from build123d import *

# Parameters (mm, degrees)
SKETCH_1_W      = 10.3
SKETCH_1_H      = 10.3
EXTRUDE_1_DEPTH = 100


with BuildPart() as part:
    # 草图1 → 凸台-拉伸1 (new body)
    with BuildSketch(Plane.XY):
        with BuildLine():
            Line((-3.371587854, 9.357012623), (-6.271587854, 9.357012623))
            Line((-6.271587854, 9.357012623), (-6.271587854, 17.757012623))
            Line((-6.271587854, 17.757012623), (-3.871587854, 17.757012623))
            ThreePointArc((-3.871587854, 17.757012623), (-3.518034464, 17.903459232), (-3.371587854, 18.257012623))
            Line((-3.371587854, 18.257012623), (-3.371587854, 20.257012623))
            ThreePointArc((-3.371587854, 20.257012623), (-3.518034464, 20.610566013), (-3.871587854, 20.757012623))
            Line((-3.871587854, 20.757012623), (-18.771587854, 20.757012623))
            ThreePointArc((-18.771587854, 20.757012623), (-19.125141245, 20.610566013), (-19.271587854, 20.257012623))
            Line((-19.271587854, 20.257012623), (-19.271587854, 5.357012623))
            ThreePointArc((-19.271587854, 5.357012623), (-19.125141245, 5.003459232), (-18.771587854, 4.857012623))
            Line((-18.771587854, 4.857012623), (-16.771587854, 4.857012623))
            ThreePointArc((-16.771587854, 4.857012623), (-16.418034464, 5.003459232), (-16.271587854, 5.357012623))
            Line((-16.271587854, 5.357012623), (-16.271587854, 7.757012623))
            Line((-16.271587854, 7.757012623), (-7.871587854, 7.757012623))
            Line((-7.871587854, 7.757012623), (-7.871587854, 4.857012623))
            Line((-7.871587854, 4.857012623), (-6.641587854, 6.087012623))
            Line((-6.641587854, 6.087012623), (-6.641587854, -4.572987377))
            Line((-6.641587854, -4.572987377), (-7.871587854, -3.342987377))
            Line((-7.871587854, -3.342987377), (-7.871587854, -6.242987377))
            Line((-7.871587854, -6.242987377), (-16.271587854, -6.242987377))
            Line((-16.271587854, -6.242987377), (-16.271587854, -3.842987377))
            ThreePointArc((-16.271587854, -3.842987377), (-16.418034464, -3.489433987), (-16.771587854, -3.342987377))
            Line((-16.771587854, -3.342987377), (-18.771587854, -3.342987377))
            ThreePointArc((-18.771587854, -3.342987377), (-19.125141245, -3.489433987), (-19.271587854, -3.842987377))
            Line((-19.271587854, -3.842987377), (-19.271587854, -18.742987377))
            ThreePointArc((-19.271587854, -18.742987377), (-19.125141245, -19.096540768), (-18.771587854, -19.242987377))
            Line((-18.771587854, -19.242987377), (-3.871587854, -19.242987377))
            ThreePointArc((-3.871587854, -19.242987377), (-3.518034464, -19.096540768), (-3.371587854, -18.742987377))
            Line((-3.371587854, -18.742987377), (-3.371587854, -16.742987377))
            ThreePointArc((-3.371587854, -16.742987377), (-3.518034464, -16.389433987), (-3.871587854, -16.242987377))
            Line((-3.871587854, -16.242987377), (-6.271587854, -16.242987377))
            Line((-6.271587854, -16.242987377), (-6.271587854, -7.842987377))
            Line((-6.271587854, -7.842987377), (-3.371587854, -7.842987377))
            Line((-3.371587854, -7.842987377), (-4.601587854, -6.612987377))
            Line((-4.601587854, -6.612987377), (6.058412146, -6.612987377))
            Line((6.058412146, -6.612987377), (4.828412146, -7.842987377))
            Line((4.828412146, -7.842987377), (7.728412146, -7.842987377))
            Line((7.728412146, -7.842987377), (7.728412146, -16.242987377))
            Line((7.728412146, -16.242987377), (5.328412146, -16.242987377))
            ThreePointArc((5.328412146, -16.242987377), (4.974858755, -16.389433987), (4.828412146, -16.742987377))
            Line((4.828412146, -16.742987377), (4.828412146, -18.742987377))
            ThreePointArc((4.828412146, -18.742987377), (4.974858755, -19.096540768), (5.328412146, -19.242987377))
            Line((5.328412146, -19.242987377), (20.228412146, -19.242987377))
            ThreePointArc((20.228412146, -19.242987377), (20.581965536, -19.096540768), (20.728412146, -18.742987377))
            Line((20.728412146, -18.742987377), (20.728412146, -3.842987377))
            ThreePointArc((20.728412146, -3.842987377), (20.581965536, -3.489433987), (20.228412146, -3.342987377))
            Line((20.228412146, -3.342987377), (18.228412146, -3.342987377))
            ThreePointArc((18.228412146, -3.342987377), (17.874858755, -3.489433987), (17.728412146, -3.842987377))
            Line((17.728412146, -3.842987377), (17.728412146, -6.242987377))
            Line((17.728412146, -6.242987377), (9.328412146, -6.242987377))
            Line((9.328412146, -6.242987377), (9.328412146, -3.342987377))
            Line((9.328412146, -3.342987377), (8.098412146, -4.572987377))
            Line((8.098412146, -4.572987377), (8.098412146, 6.087012623))
            Line((8.098412146, 6.087012623), (9.328412146, 4.857012623))
            Line((9.328412146, 4.857012623), (9.328412146, 7.757012623))
            Line((9.328412146, 7.757012623), (17.728412146, 7.757012623))
            Line((17.728412146, 7.757012623), (17.728412146, 5.357012623))
            ThreePointArc((17.728412146, 5.357012623), (17.874858755, 5.003459232), (18.228412146, 4.857012623))
            Line((18.228412146, 4.857012623), (20.228412146, 4.857012623))
            ThreePointArc((20.228412146, 4.857012623), (20.581965536, 5.003459232), (20.728412146, 5.357012623))
            Line((20.728412146, 5.357012623), (20.728412146, 20.257012623))
            ThreePointArc((20.728412146, 20.257012623), (20.581965536, 20.610566013), (20.228412146, 20.757012623))
            Line((20.228412146, 20.757012623), (5.328412146, 20.757012623))
            ThreePointArc((5.328412146, 20.757012623), (4.974858755, 20.610566013), (4.828412146, 20.257012623))
            Line((4.828412146, 20.257012623), (4.828412146, 18.257012623))
            ThreePointArc((4.828412146, 18.257012623), (4.974858755, 17.903459232), (5.328412146, 17.757012623))
            Line((5.328412146, 17.757012623), (7.728412146, 17.757012623))
            Line((7.728412146, 17.757012623), (7.728412146, 9.357012623))
            Line((7.728412146, 9.357012623), (4.828412146, 9.357012623))
            Line((4.828412146, 9.357012623), (6.058412146, 8.127012623))
            Line((6.058412146, 8.127012623), (-4.601587854, 8.127012623))
            Line((-4.601587854, 8.127012623), (-3.371587854, 9.357012623))
        make_face()
        with Locations((-12.421587854, 13.907012623)):
            Rectangle(SKETCH_1_W, SKETCH_1_H, mode=Mode.SUBTRACT)
        with Locations((13.878412146, 13.907012623)):
            Rectangle(SKETCH_1_W, SKETCH_1_H, mode=Mode.SUBTRACT)
        with Locations((-12.421587854, -12.392987377)):
            Rectangle(SKETCH_1_W, SKETCH_1_H, mode=Mode.SUBTRACT)
        with Locations((13.878412146, -12.392987377)):
            Rectangle(SKETCH_1_W, SKETCH_1_H, mode=Mode.SUBTRACT)
        with BuildLine():
            Line((-5.448612368, 5.519823574), (-3.44279625, 3.514007457))
            ThreePointArc((-3.44279625, 3.514007457), (-3.890985517, 2.670429785), (-4.17056734, 1.757012623))
            Line((-4.17056734, 1.757012623), (-5.187667637, 1.757012623))
            ThreePointArc((-5.187667637, 1.757012623), (-5.271587854, 0.757012623), (-5.187667637, -0.242987377))
            Line((-5.187667637, -0.242987377), (-4.17056734, -0.242987377))
            ThreePointArc((-4.17056734, -0.242987377), (-3.890985517, -1.156404539), (-3.44279625, -1.999982211))
            Line((-3.44279625, -1.999982211), (-5.448612368, -4.005798329))
            ThreePointArc((-5.448612368, -4.005798329), (-4.787020747, -4.758420271), (-4.034398805, -5.420011891))
            Line((-4.034398805, -5.420011891), (-2.028582688, -3.414195774))
            ThreePointArc((-2.028582688, -3.414195774), (-1.185005016, -3.86238504), (-0.271587854, -4.141966863))
            Line((-0.271587854, -4.141966863), (-0.271587854, -5.15906716))
            ThreePointArc((-0.271587854, -5.15906716), (0.728412146, -5.242987377), (1.728412146, -5.15906716))
            Line((1.728412146, -5.15906716), (1.728412146, -4.141966863))
            ThreePointArc((1.728412146, -4.141966863), (2.641829308, -3.86238504), (3.48540698, -3.414195774))
            Line((3.48540698, -3.414195774), (5.491223097, -5.420011891))
            ThreePointArc((5.491223097, -5.420011891), (6.243845039, -4.758420271), (6.905436659, -4.005798329))
            Line((6.905436659, -4.005798329), (4.899620542, -1.999982211))
            ThreePointArc((4.899620542, -1.999982211), (5.347809808, -1.156404539), (5.627391631, -0.242987377))
            Line((5.627391631, -0.242987377), (6.644491929, -0.242987377))
            ThreePointArc((6.644491929, -0.242987377), (6.728412146, 0.757012623), (6.644491929, 1.757012623))
            Line((6.644491929, 1.757012623), (5.627391631, 1.757012623))
            ThreePointArc((5.627391631, 1.757012623), (5.347809808, 2.670429785), (4.899620542, 3.514007457))
            Line((4.899620542, 3.514007457), (6.905436659, 5.519823574))
            ThreePointArc((6.905436659, 5.519823574), (6.243845039, 6.272445516), (5.491223097, 6.934037136))
            Line((5.491223097, 6.934037136), (3.48540698, 4.928221019))
            ThreePointArc((3.48540698, 4.928221019), (2.641829308, 5.376410285), (1.728412146, 5.655992108))
            Line((1.728412146, 5.655992108), (1.728412146, 6.673092406))
            ThreePointArc((1.728412146, 6.673092406), (0.728412146, 6.757012623), (-0.271587854, 6.673092406))
            Line((-0.271587854, 6.673092406), (-0.271587854, 5.655992108))
            ThreePointArc((-0.271587854, 5.655992108), (-1.185005016, 5.376410285), (-2.028582688, 4.928221019))
            Line((-2.028582688, 4.928221019), (-4.034398805, 6.934037136))
            ThreePointArc((-4.034398805, 6.934037136), (-4.787020747, 6.272445516), (-5.448612368, 5.519823574))
        make_face(mode=Mode.SUBTRACT)
    extrude(amount=EXTRUDE_1_DEPTH)


solid = part.part
Here's how the part is built. I have some questions about the finished solid (model axes, mm). A direction names the side the tool comes from. Round coordinates to 2 decimals unless told otherwise and drop trailing zeros. Loops run counter-clockwise (first coordinate to the right, second up) from the corner with the lowest first, then second, coordinate; pieces in that order, holes last.
1. If we section it at B-B on x = -9.5: Write out the boundary of the cut face in (y, z).
Answer list:
outline: (-19.24, 0) - (-17.54, 0) - (-17.54, 100) - (-19.24, 100) - close; (-7.24, 0) - (-6.24, 0) - (-6.24, 100) - (-7.24, 100) - close; (7.76, 0) - (8.76, 0) - (8.76, 100) - (7.76, 100) - close; (19.06, 0) - (20.76, 0) - (20.76, 100) - (19.06, 100) - close
2. If we section it at C-C on z = 47: Count the separate pieces of the cut face and the enclosed holes in it, plus the area to 3 significant figures.
Answer list:
separate pieces: 1
enclosed holes: 5
area: 450 mm2
3. For P1, Ø5, axis at x = 2.5, z = 11.5, coming from the +Y side; P2, Ø8.5, axis at y = 2.5, z = 45.5, coming from the -X side, each with a flat end and sliding along its axis, tell me the tip position at first contact or that it passes through.
Answer list:
P1: stops at y = 20.63
P2: stops at x = -19.27
4. If I drill on line 1 along Y through (x, z) = (-6, 43.5); line 2 along Y through (x, z) = (16.5, 37); line 3 along X through (y, z) = (-9.5, 22), over which ranges is the centre line in solid material (lowest first)?
Answer list:
line 1: y = -19.24 to -16.24, -7.84 to 9.36, 17.76 to 20.76
line 2: y = -19.24 to -17.54, -7.24 to -6.24, 7.76 to 8.76, 19.06 to 20.76
line 3: x = -19.27 to -17.57, -7.27 to -6.27, 7.73 to 8.73, 19.03 to 20.73
5. Which directions (+Z, -Z, +X, -X, +Y, -Y) give clear straight access to the entire face, cutting with the end or side of a thin tool? Please do faces 3 (the face through (19.028, -12, 49)), 4 (the face through (-18, 4.857, 49)), 5 (the face through (19, -3.343, 49)).
Answer list:
face 3: +Z, -Z
face 4: +Z, -Z, -X
face 5: +Z, -Z, +X
6. If we section it at A-A on y = -13: Write out the boundary of the cut face in (x, z), plus the area to 3 significant figures.
Answer list:
outline: (-19.27, 0) - (-17.57, 0) - (-17.57, 100) - (-19.27, 100) - close; (-7.27, 0) - (-6.27, 0) - (-6.27, 100) - (-7.27, 100) - close; (7.73, 0) - (8.73, 0) - (8.73, 100) - (7.73, 100) - close; (19.03, 0) - (20.73, 0) - (20.73, 100) - (19.03, 100) - close
area: 540 mm2
7. We'd pull the mould along Y, two halves only. Please class faces 1 (the face through (20.728, 13, 49)), 2 (the face through (-5, -16.243, 49)): +Y half, -Y half, draft (parallel to the pull), parting line (faces both ways), or undercut.
Answer list:
face 1: draft
face 2: undercut
